Verification items for the finished model (mm, model axes). Coordinates: 2 decimals unless noted, no trailing zeros. Loops run counter-clockwise (first coordinate to the right, second up) from the corner with the lowest first, then second, coordinate; pieces in that order, holes last.
Q1. Material ranges on probe 1 along Z at (x, y) = (70, 12.25); probe 2 along Y at (x, z) = (7.5, -23); probe 3 along Y at (x, z) = (32.5, -172.5), recorded low to high.
Q2. Sectioned sample at A-A (x = 35). Count the separate pieces of the cut face and the enclosed holes in it, then the cut area to 3 significant figures.
Q3. Sectioned sample at C-C (z = -142.5). Enter the section's corners in (x, y), then the cut area to 4 significant figures.
Q4. Go/stop test with flat-tipped pins: P1, Ø5, axis at x = 36, y = 6.5, coming from the -Z side (1 decimal); P2, Ø12, axis at x = 74.5, z = -142.5, coming from the +Y side; P3, Ø9.5, axis at x = 44.5, y = 13, coming from the +Z side. Record where each tip stops, or that it passes through.
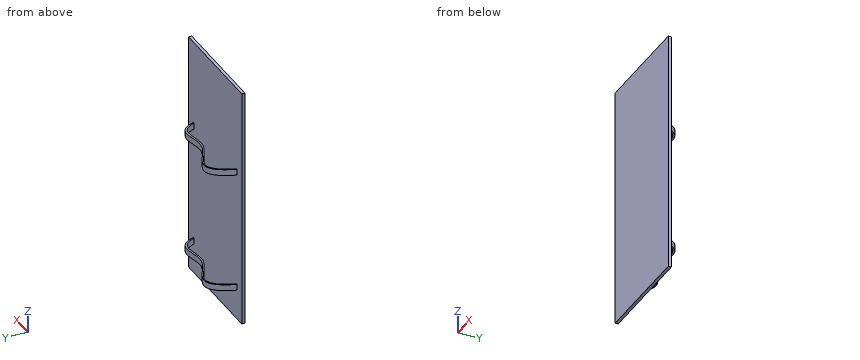
```python
from build123d import *

# Parameters (mm, degrees)
SKETCH1_W           = 85
SKETCH1_H           = 200
BOSS_EXTRUDE1_DEPTH = 2.5
BOSS_EXTRUDE3_DEPTH = 5
LPATTERN1_COUNT     = 2
LPATTERN1_PITCH     = 100


with BuildPart() as part:
    # Sketch1 → Boss-Extrude1 (new body)
    with BuildSketch(Plane(origin=(0, 0, 0), x_dir=(1, 0, 0), z_dir=(0, 1, 0))):
        with Locations((42.5, 100)):
            Rectangle(SKETCH1_W, SKETCH1_H)
    extrude(amount=BOSS_EXTRUDE1_DEPTH)

    # Sketch3 → Boss-Extrude3 (add)
    with BuildSketch(Plane(origin=(0, 0, -175), x_dir=(-1, 0, 0), z_dir=(0, 0, -1))):
        with BuildLine():
            Line((-77.5, 2.5), (-76.450132059, 2.5))
            add(Edge.make_bspline(
                [(-76.450132059, 2.5), (-76.352037023, 2.813155952), (-76.141653781, 3.448774979), (-75.712920238, 4.60640845), (-75.141711698, 5.914949297), (-74.412627596, 7.255247487), (-73.387535674, 8.763975464), (-72.02254847, 10.166201705), (-70.263673421, 11.232606933), (-68.348427729, 11.819901852), (-65.552395249, 12.079641822), (-61.64077912, 11.600566429), (-56.547104343, 10.479098709), (-52.154053067, 9.794168924), (-48.61006882, 9.853555219), (-45.138239485, 10.48501356), (-41.055154093, 12.11371223), (-36.455574443, 14.746231277), (-32.098424566, 17.443496584), (-27.955000453, 19.605965858), (-24.067408798, 20.651525579), (-21.036519902, 20.26070597), (-18.540531077, 18.923836601), (-16.603695352, 17.289307939), (-14.606368482, 14.925983967), (-12.900683609, 12.280076139), (-11.514973715, 9.719991389), (-10.466169356, 7.570851399), (-9.58244987, 5.576333061), (-8.874263801, 3.865936613), (-8.511972004, 2.951657976), (-8.336705052, 2.5)],
                knots=[0, 0, 0, 0, 0.0078125, 0.015625, 0.03125, 0.046875, 0.0625, 0.09375, 0.125, 0.15625, 0.1875, 0.25, 0.3125, 0.375, 0.40625, 0.4375, 0.5, 0.5625, 0.625, 0.6875, 0.75, 0.8125, 0.84375, 0.875, 0.90625, 0.9375, 0.953125, 0.96875, 0.984375, 0.9921875, 1, 1, 1, 1], degree=3))
            Line((-8.336705052, 2.5), (-7.5, 2.5))
            add(Edge.make_bspline(
                [(-77.5, 2.5), (-72.458418192, 21.091936155), (-41.386339311, -5.263286213), (-20.750377369, 38.155046939), (-7.5, 2.5)],
                knots=[0, 0, 0, 0, 0.411408499, 1, 1, 1, 1], degree=3))
        make_face()
    boss_extrude3 = extrude(amount=-BOSS_EXTRUDE3_DEPTH)

    # LPattern1: Boss-Extrude3 ×2
    with Locations(*[(0, 0, i * LPATTERN1_PITCH) for i in range(1, LPATTERN1_COUNT)]):
        add(boss_extrude3)


solid = part.part
```
Geometry check:
1. probe 1: z = -175 to -170, -75 to -70
1. probe 2: y = 0 to 2.5
1. probe 3: y = 0 to 2.5, 17.14 to 18.3
2. separate pieces: 3
2. enclosed holes: 0
2. area: 512 mm2
3. outline: (0, 0) - (85, 0) - (85, 2.5) - (0, 2.5) - close
3. area: 212.5 mm2
4. P1: passes through
4. P2: stops at y = 2.5
4. P3: stops at z = -70
